```python
from build123d import *

# Parameters (mm, degrees)
SKETCH1_W           = 38.1
SKETCH1_H           = 38.1
SKETCH1_W_2         = 31.75
SKETCH1_H_2         = 31.75
BOSS_EXTRUDE1_DEPTH = 1828.8
SKETCH2_R           = 6.35
CUT_EXTRUDE1_DEPTH  = 38.1


with BuildPart() as part:
    # Sketch1 → Boss-Extrude1 (new body)
    with BuildSketch(Plane.XY):
        Rectangle(SKETCH1_W, SKETCH1_H)
        Rectangle(SKETCH1_W_2, SKETCH1_H_2, mode=Mode.SUBTRACT)
    extrude(amount=-BOSS_EXTRUDE1_DEPTH)

    # Sketch2 → Cut-Extrude1 (cut)
    with BuildSketch(Plane.ZY.offset(19.05)):
        with Locations((-25.4, 0)):
            Circle(SKETCH2_R)
    extrude(amount=-CUT_EXTRUDE1_DEPTH, mode=Mode.SUBTRACT)


solid = part.part
```
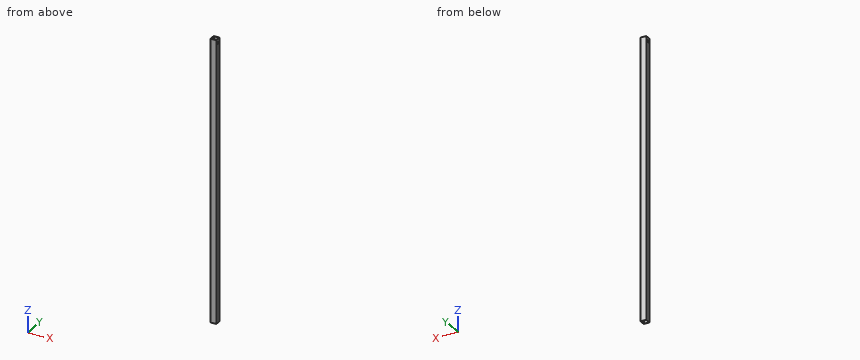
Input: part model. Units: mm. Frame: model coordinates. Round coordinates to 2 decimals unless told otherwise and drop trailing zeros. Order: outer loops, then holes, each group sorted by start corner. A loop starts at its lowest first (then second) coordinate and runs counter-clockwise, first axis right, second up. Notation, with made-up numbers: (75, 43) - (122, 43) arc R21 ccw to (122, 49) - close; hole circle Ø4 at (67.5, -33.5). An arc over 180 degrees is marked (long way). Answer in a Markdown table with one row per item.
Item 1: Line query: line 1 (Y direction, x = 15.5, z = -1722) (3 decimals); line 2 (Y direction, x = -17.1, z = -25.4). Output: solid intervals per line, ascending.
Model answer:
| item | result |
|---|---|
| line 1 | y = -19.05 to -15.875, 15.875 to 19.05 |
| line 2 | y = -19.05 to -6.35, 6.35 to 19.05 |
Item 2: Pin query (flat end, axial travel): pin 1 (11.5 mm diameter, centred on y = 0, z = -25.4, fed in from +X). Return the tip coordinate at first contact, or that it passes through.
Model answer:
| item | result |
|---|---|
| pin 1 | passes through |
Item 3: Section query C-C (z = -873). Return the cut outline in (x, y) (3 decimals).
Model answer:
| item | result |
|---|---|
| outline | (-19.05, -19.05) - (19.05, -19.05) - (19.05, 19.05) - (-19.05, 19.05) - close; hole (-15.875, -15.875) - (15.875, -15.875) - (15.875, 15.875) - (-15.875, 15.875) - close |
Item 4: Section query B-B (y = 0). Return the cut outline in (x, z) (3 decimals), then the cut area to 3 significant figures.
Model answer:
| item | result |
|---|---|
| outline | (-19.05, -1828.8) - (-15.875, -1828.8) - (-15.875, -31.75) - (-19.05, -31.75) - close; (-19.05, -19.05) - (-15.875, -19.05) - (-15.875, 0) - (-19.05, 0) - close; (15.875, -1828.8) - (19.05, -1828.8) - (19.05, -31.75) - (15.875, -31.75) - close; (15.875, -19.05) - (19.05, -19.05) - (19.05, 0) - (15.875, 0) - close |
| area | 11,500 mm² |
Item 5: Section query A-A (x = 1). Return the cut outline in (y, z) (3 decimals).
Model answer:
| item | result |
|---|---|
| outline | (-19.05, -1828.8) - (-15.875, -1828.8) - (-15.875, 0) - (-19.05, 0) - close; (15.875, -1828.8) - (19.05, -1828.8) - (19.05, 0) - (15.875, 0) - close |
